CAD build for the part. Positions are in the model's coordinates, mm. A direction names the side the tool comes from. Round coordinates to 2 decimals unless told otherwise and drop trailing zeros. Order: outer loops, then holes, each group sorted by start corner. A loop starts at its lowest first (then second) coordinate and runs counter-clockwise, first axis right, second up. Notation, with made-up numbers: (58.25, 30) - (69.25, 30) arc R18 ccw to (69.25, 52) - close; hole circle Ø5 at (7, -38). An arc over 180 degrees is marked (long way). Write item = value, one per line.
Autodesk Inventor part; units mm, degrees
ref_plane "YZ Plane" through (0, 0, 0) normal (1, 0, 0) x (0, 1, 0)
ref_plane "XZ Plane" through (0, 0, 0) normal (0, 1, 0) x (-1, 0, 0)
ref_plane "XY Plane" through (0, 0, 0) normal (0, 0, 1) x (1, 0, 0)
sketch "Sketch1" plane through (0, 0, 0) normal (0, 0, 1) x (1, 0, 0)
  line L0 (0, 0) -> (66.675, 0)
  line L1 (66.675, 0) -> (66.675, -12.7)
  line L2 (66.675, -12.7) -> (0, -12.7)
  line L3 (0, -12.7) -> (0, 0)
  dimension "d0" = 66.675
  dimension "d1" = 12.7
extrude "Extrusion1" add sketch "Sketch1" along normal blind 3.175
fillet "Fillet1" radius 0.635 8 edges at (33.3375, 0, 0) (66.675, -6.35, 0) (66.675, 0, 1.5875) (33.3375, -12.7, 0) (66.675, -12.7, 1.5875) (0, -6.35, 0) (0, -12.7, 1.5875) (0, 0, 1.5875)
sketch "Sketch2" plane through (0, 0, 3.175) normal (0, 0, 1) x (1, 0, 0)
  line L0 (66.04, 0) -> (0.635, 0)
  line L1 (0.635, -12.7) -> (66.04, -12.7)
  line L2 (9.525, 0) -> (57.15, 0)
  line L3 (57.15, 0) -> (57.15, -12.7)
  line L4 (57.15, -12.7) -> (9.525, -12.7)
  line L5 (9.525, -12.7) -> (9.525, 0)
  line L6 (66.675, -12.065) -> (66.675, -0.635)
  point P0 (0, 0)
  dimension "d5" = 47.625
  dimension "d6" = 9.525
extrude "Extrusion2" cut sketch "Sketch2" against normal blind 1.397
sketch "Sketch3" plane through (0, 0, 3.175) normal (0, 0, 1) x (1, 0, 0)
  line L0 (66.04, -0.635) -> (0.635, -0.635)
  line L1 (0.635, -12.065) -> (66.04, -12.065)
  line L2 (5.842, -1.27) -> (7.62, -1.27)
  line L3 (7.62, -1.27) -> (7.62, -11.43)
  line L4 (7.62, -11.43) -> (5.842, -11.43)
  line L5 (5.842, -11.43) -> (5.842, -1.27)
  line L6 (9.525, -12.7) -> (9.525, 0)
  line L7 (7.112, -1.101) -> (5.842, -11.4757)
  line L8 (5.842, -11.4757) -> (8.89, -11.4757)
  line L9 (8.89, -11.4757) -> (7.62, -21.8503)
  line L10 (9.525, 0) -> (0.635, 0)
  line L11 (0.635, -12.7) -> (9.525, -12.7)
  point P0 (0, 0)
  dimension "d9" = 1.778
  dimension "d52" = 1.27
  dimension "d53" = 1.27
  dimension "d56" = 1.905
extrude "Extrusion3" add sketch "Sketch3" along normal blind 3.81 contours L4 L5 L2 L7 | L7 L2 L3 L4
sketch "Sketch5" plane through (0, 0, 3.175) normal (0, 0, 1) x (1, 0, 0)
  line L0 (66.04, -0.635) -> (0.635, -0.635)
  line L1 (0.635, -12.065) -> (66.04, -12.065)
  line L2 (59.055, -1.27) -> (60.833, -1.27)
  line L3 (60.833, -1.27) -> (60.833, -11.43)
  line L4 (60.833, -11.43) -> (59.055, -11.43)
  line L5 (59.055, -11.43) -> (59.055, -1.27)
  line L6 (57.15, 0) -> (57.15, -12.7)
  line L7 (66.04, 0) -> (57.15, 0)
  line L8 (57.15, -12.7) -> (66.04, -12.7)
  point P0 (0, 0)
  dimension "d21" = 1.778
  dimension "d54" = 1.27
  dimension "d55" = 1.27
  dimension "d57" = 1.905
extrude "Extrusion5" add sketch "Sketch5" along normal blind 3.175
sketch "Sketch6" plane through (59.055, -1.27, 3.175) normal (0, 1, 0) x (1, 0, 0)
  line L0 (0, 0) -> (1.778, 0)
  line L1 (1.016, -1.524) -> (1.016, 0)
  line L2 (1.016, 0) -> (0, 0)
  line L3 (0, 0) -> (0, -1.524)
  line L4 (0, 0) -> (0, -3.175)
  line L5 (0, 0) -> (1.016, 0)
  line L6 (1.016, 0) -> (1.016, -1.524)
  line L7 (1.016, -1.524) -> (0, -1.524)
  line L8 (0, -1.524) -> (0, 0)
  point P0 (-59.055, 3.175)
  point P1 (0, -1.524)
  dimension "d29" = 1.016
  dimension "d51" = 1.524
extrude "Extrusion6" cut sketch "Sketch6" against normal through all
sketch "Sketch7" plane through (0, 0, 1.778) normal (0, 0, 1) x (1, 0, 0)
  line L0 (9.525, -12.7) -> (9.525, 0)
  line L1 (57.15, 0) -> (57.15, -12.7)
  line L2 (9.525, -5.9055) -> (57.15, -5.9055)
  line L3 (57.15, -5.9055) -> (57.15, -6.7945)
  line L4 (57.15, -6.7945) -> (9.525, -6.7945)
  line L5 (9.525, -6.7945) -> (9.525, -5.9055)
  line L6 (9.525, 0) -> (57.15, 0)
  point P0 (0, 0)
  dimension "d33" = 0.889
  dimension "d34" = 5.9055
extrude "Extrusion7" add sketch "Sketch7" along normal blind 1.016 contours L0 L2 L1 L4
sketch "Sketch8" plane through (5.842, -1.27, 3.175) normal (0, 1, 0) x (1, 0, 0)
  line L0 (0, 0) -> (1.778, 0)
  line L1 (1.778, 0) -> (0.762, 0)
  line L2 (0.762, 0) -> (0.762, -1.524)
  line L3 (0.762, -1.524) -> (1.778, -1.524)
  line L4 (1.778, -1.524) -> (1.778, 0)
  point P0 (-5.842, 3.175)
  dimension "d38" = 1.016
  dimension "d39" = 1.524
extrude "Extrusion8" cut sketch "Sketch8" against normal through all
chamfer "Chamfer3" distance 1.778 angle 30 1 edges at (7.62, -6.35, 6.985) measured on face at (6.4347, -4.6567, 6.985)
fillet "Fillet4" radius 0.3175 1 edges at (7.62, -6.35, 5.959)
chamfer "Chamfer4" distance 1.778 angle 25 1 edges at (59.055, -6.35, 6.35) measured on face at (59.6477, -4.6567, 6.35)
fillet "Fillet5" radius 0.3175 1 edges at (59.055, -6.35, 5.5214)
properties part number "ClipMale"
(1) Pull direction Z, two halves, no side cores. Call faces 4 (the flat face through (6.604, -6, 4)), 5 (the flat face through (0, -6, 2)), 6 (the flat face through (60.02, -6.42, 5.97)), 7 (the flat face through (33, -6, 0)): released by +Z, released by -Z, zero draft, split by the parting line, or undercut.
Solved:
face_4 = undercut
face_5 = zero draft
face_6 = released by +Z
face_7 = released by -Z
(2) Drop flat-ended pins along their axis: pin 1 (2 mm diameter, centred on x = 60, z = 4.5, fed in from +Y); pin 2 (4.5 mm diameter, centred on x = 29.5, y = -2.5, fed in from +Z); pin 3 (1 mm diameter, centred on x = 29.5, z = 2.5, fed in from +Y); pin 4 (1.1 mm diameter, centred on x = 31.5, z = 2, fed in from -Y). Give the stop position or say it passes through.
Solved:
pin_1 = -1.27
pin_2 = 1.78
pin_3 = -5.91
pin_4 = -12.7
(3) Probe line 1 along X through (y, z) = (-10.5, 3.5); line 2 along X through (y, z) = (-4, 4.75) (3 decimals); line 3 along Y through (x, z) = (25.5, 2). List the from-to ranges inside material, lowest first.
Solved:
line_1 = 5.84 to 6.6, 60.07 to 60.83
line_2 = 5.842 to 7.62, 59.055 to 60.833
line_3 = -6.79 to -5.91
(4) Band-saw the part on B-B on x = 51. List the corners of the cut face in (y, z) (1 decimal), plus the area to 3 significant figures.
Solved:
outline = (-12.7, 0.6) arc R0.6 ccw to (-12.1, 0) - (-0.6, 0) arc R0.6 ccw to (0, 0.6) - (0, 1.8) - (-5.9, 1.8) - (-5.9, 2.8) - (-6.8, 2.8) - (-6.8, 1.8) - (-12.7, 1.8) - close
area = 23.3 mm²
(5) Tool access for faces 1 (the flat face through (7, -11.43, 5)), 2 (the flat face through (9.525, -6, 3)), 3 (the flat face through (33, -10, 1.778)): list every direction of +Z, -Z, +X, -X, +Y, -Y with a clear straight run to the whole face (end or side of a thin tool).
Solved:
face_1 = +Z, +X, -X, -Y
face_2 = +Z
face_3 = +Z, -Y
